```python
from build123d import *

# Parameters (mm, degrees)
F0_W     = 25.4
F0_H     = 50.8
F1_DEPTH = 1800
F2_R     = 7.5
F3_DEPTH = 25.4
F4_R     = 7.5
F5_DEPTH = 25.4


with BuildPart() as f1:
    # F0 (on Right) → F1 (new body)
    with BuildSketch(Plane.YZ):
        Rectangle(F0_W, F0_H)
        with BuildLine():
            Line((-8.2, 22.9), (8.2, 22.9))
            ThreePointArc((8.2, 22.9), (9.614214, 22.314214), (10.2, 20.9))
            Line((10.2, 20.9), (10.2, -20.9))
            ThreePointArc((10.2, -20.9), (9.614214, -22.314214), (8.2, -22.9))
            Line((8.2, -22.9), (-8.2, -22.9))
            ThreePointArc((-8.2, -22.9), (-9.614214, -22.314214), (-10.2, -20.9))
            Line((-10.2, -20.9), (-10.2, 20.9))
            ThreePointArc((-10.2, 20.9), (-9.614214, 22.314214), (-8.2, 22.9))
        make_face(mode=Mode.SUBTRACT)
    extrude(amount=F1_DEPTH)

    # F2 (on face) → F3 (cut, through all)
    with BuildSketch(Plane.XZ.offset(12.7)):
        with Locations((1760, 0)):
            Circle(F2_R)
    extrude(amount=-F3_DEPTH, mode=Mode.SUBTRACT)

    # F4 (on face) → F5 (cut, through all)
    with BuildSketch(Plane.XZ.offset(12.7)):
        with Locations((40, 0)):
            Circle(F4_R)
        with Locations((80, 0)):
            Circle(F4_R)
        with Locations((120, 0)):
            Circle(F4_R)
        with Locations((160, 0)):
            Circle(F4_R)
        with Locations((200, 0)):
            Circle(F4_R)
    extrude(amount=-F5_DEPTH, mode=Mode.SUBTRACT)


solid = f1.part
```
Work out the finished part from the listing and answer in its coordinate system (mm). A direction names the side the tool comes from. Give positions to 0.01 mm unless a question says otherwise; leave off trailing zeros. Write each loop counter-clockwise with the first axis right and the second up, starting at its lowest first coordinate (ties: lowest second). Pieces come first, ordered by that corner, then holes.
(1) A flat-ended cylindrical pin translates along its axis: pin 1 Ø9 at (x, z) = (160, 0) entering from +Y. Find the tip coordinate at first contact, or state that the pin passes through.
Final values:
pin 1: passes through
(2) The part is cut by section B-B on x = 244.5. Write down the section's boundary in (y, z), plus the area to 3 significant figures.
Final values:
outline: (-12.7, -25.4) - (12.7, -25.4) - (12.7, 25.4) - (-12.7, 25.4) - close; hole (-10.2, -20.9) arc R2 ccw to (-8.2, -22.9) - (8.2, -22.9) arc R2 ccw to (10.2, -20.9) - (10.2, 20.9) arc R2 ccw to (8.2, 22.9) - (-8.2, 22.9) arc R2 ccw to (-10.2, 20.9) - close
area: 359 mm2
(3) The mould has two halves that part along Z. Classify faces 1 (the flat face through (887, 10.2, 0)), 2 (the flat face through (887, 12.7, 0)): pulls with the +Z half, pulls with the -Z half, needs draft (parallel to the pull), parting line crosses it, or undercut.
Final values:
face 1: undercut
face 2: needs draft
(4) Which of the six approach directions +Z, -Z, +X, -X, +Y, -Y give full straight-line access (tool end or side, diameter ignored) to faces 3 (the flat face through (887, -10.2, 0)), 4 (the flat face through (887, -12.7, 0))?
Final values:
face 3: +X, -X
face 4: +Z, -Z, +X, -X, -Y
(5) The part is cut by section A-A on y = 3. Write down the section's boundary in (x, z), plus the area to 3 significant figures.
Final values:
outline: (0, -25.4) - (1800, -25.4) - (1800, -22.9) - (0, -22.9) - close; (0, 22.9) - (1800, 22.9) - (1800, 25.4) - (0, 25.4) - close
area: 9,000 mm2
(6) Straight lines are drawn through the part: line 1 (Z direction, x = 1266.5, y = 5); line 2 (Y direction, x = 875.5, z = -18); line 3 (Z direction, x = 1760, y = 11). For each, find the intervals that lie inside material, in ascending order.
Final values:
line 1: z = -25.4 to -22.9, 22.9 to 25.4
line 2: y = -12.7 to -10.2, 10.2 to 12.7
line 3: z = -25.4 to -7.5, 7.5 to 25.4
